Read the model definition and answer for the solid it produces. Units are mm, in the model's axes. A direction names the side the tool comes from. Round coordinates to 2 decimals unless told otherwise and drop trailing zeros. Order: outer loops, then holes, each group sorted by start corner. A loop starts at its lowest first (then second) coordinate and runs counter-clockwise, first axis right, second up. Notation, with made-up numbers: (20.5, 50.5) - (52.5, 50.5) arc R9 cw to (52.5, 65.5) - close; hole circle Ø3 at (-7, 22.5). An arc over 180 degrees is marked (long way). One line per question, with ' | ' between items. Start each with the question number.
1) Flat-ended cylindrical pins translate along their axes: pin 1 (5 mm diameter, centred on y = -81.5, z = 5, fed in from +X); pin 2 (1.5 mm diameter, centred on x = -86, z = 8, fed in from +Y); pin 3 (3 mm diameter, centred on x = 17.5, z = 6, fed in from -Y); pin 4 (3.5 mm diameter, centred on x = -61.35, y = -84.13, fed in from +Z). Find the tip coordinate at first contact, or state that the pin passes through.
2) The part is cut by section D-D, the plane y = 65.5. Give the vertices of the cut face in (x, z), plus the area to 3 significant figures.
3) Straight lines are drawn through the part: line 1 (X direction, y = 6, z = 5.5); line 2 (Y direction, x = -16.5, z = 1); line 3 (X direction, y = 87, z = 4). For each, find the intervals that lie inside material, in ascending order. Write a range as from..to.
4) The mould has two halves that part along Y. Classify faces 4 (the cylindrical face through (-124.84, 5.17, 4.93)), 5 (the flat face through (-41.355, -82, 5)), 6 (the flat face through (58, -96.132, 5)), 7 (the cylindrical face through (-144.84, 7.85, 4.93)): pulls with the +Y half, pulls with the -Y half, needs draft (parallel to the pull), parting line crosses it, or undercut.
5) The part is cut by section B-B, the plane y = 22. Give the vertices of the cut face in (x, z).
6) The part is cut by section A-A, the plane x = 21. Give the vertices of the cut face in (y, z).
7) The part is cut by section C-C, the plane z = 5.25. Give the vertices of the cut face in (x, y), plus the area to 3 significant figures.
8) For faces 1 (the flat face through (78.645, 94, 5)), 2 (the flat face through (-1, 81.068, 5)), 3 (the flat face through (-2, 61.068, 5)), determine the directions among +Z, -Z, +X, -X, +Y, -Y from which every point of the face is accessible in a straight line to the end or side of a thin tool.
from build123d import *

# Parameters (mm, degrees)
SKETCH1_R           = 1.95
BOSS_EXTRUDE1_DEPTH = 10


with BuildPart() as part:
    # Sketch1 → Boss-Extrude1 (new body)
    with BuildSketch(Plane.XY):
        with BuildLine():
            ThreePointArc((-81.354892482, 80.223597026), (-144.854892482, 6.367994666), (-81.354892482, -67.487607695))
            Line((-81.354892482, -67.487607695), (-81.354892482, -96.132005334))
            Line((-81.354892482, -96.132005334), (-41.354892482, -96.132005334))
            Line((-41.354892482, -96.132005334), (-41.354892482, -68.332005334))
            Line((-41.354892482, -68.332005334), (38.645107518, -68.332005334))
            Line((38.645107518, -68.332005334), (38.645107518, -96.132005334))
            Line((38.645107518, -96.132005334), (78.645107518, -96.132005334))
            Line((78.645107518, -96.132005334), (78.645107518, -67.487607695))
            ThreePointArc((78.645107518, -67.487607695), (142.145107518, 6.367994666), (78.645107518, 80.223597026))
            Line((78.645107518, 80.223597026), (78.645107518, 108.867994666))
            Line((78.645107518, 108.867994666), (38.645107518, 108.867994666))
            Line((38.645107518, 108.867994666), (38.645107518, 81.067994666))
            Line((38.645107518, 81.067994666), (-41.354892482, 81.067994666))
            Line((-41.354892482, 81.067994666), (-41.354892482, 108.867994666))
            Line((-41.354892482, 108.867994666), (-81.354892482, 108.867994666))
            Line((-81.354892482, 108.867994666), (-81.354892482, 80.223597026))
        make_face()
        with Locations((-136.354892482, 6.367994666)):
            Circle(SKETCH1_R, mode=Mode.SUBTRACT)
        with Locations((133.645107518, 6.367994666)):
            Circle(SKETCH1_R, mode=Mode.SUBTRACT)
        with BuildLine():
            Line((-70.154892482, 61.067994666), (67.445107518, 61.067994666))
            ThreePointArc((67.445107518, 61.067994666), (122.145107518, 6.367994666), (67.445107518, -48.332005334))
            Line((67.445107518, -48.332005334), (-70.154892482, -48.332005334))
            ThreePointArc((-70.154892482, -48.332005334), (-124.854892482, 6.367994666), (-70.154892482, 61.067994666))
        make_face(mode=Mode.SUBTRACT)
        with Locations((-61.354892482, 96.867994666)):
            Circle(SKETCH1_R, mode=Mode.SUBTRACT)
        with Locations((58.645107518, 96.867994666)):
            Circle(SKETCH1_R, mode=Mode.SUBTRACT)
        with Locations((-61.354892482, -84.132005334)):
            Circle(SKETCH1_R, mode=Mode.SUBTRACT)
        with Locations((58.645107518, -84.132005334)):
            Circle(SKETCH1_R, mode=Mode.SUBTRACT)
    extrude(amount=BOSS_EXTRUDE1_DEPTH)


solid = part.part
Values:
1) pin 1: stops at x = 78.65 | pin 2: stops at y = 79.53 | pin 3: stops at y = -68.33 | pin 4: passes through
2) outline: (-115.8, 0) - (113.09, 0) - (113.09, 10) - (-115.8, 10) - close | area: 2,290 mm^2
3) line 1: x = -144.85..-138.27, -134.44..-124.85, 122.14..131.73, 135.56..142.14 | line 2: y = -68.33..-48.33, 61.07..81.07 | line 3: x = -81.35..-41.35, 38.65..78.65
4) face 4: undercut | face 5: needs draft | face 6: pulls with the -Y half | face 7: parting line crosses it
5) outline: (-143.2, 0) - (-122.57, 0) - (-122.57, 10) - (-143.2, 10) - close; (119.86, 0) - (140.49, 0) - (140.49, 10) - (119.86, 10) - close
6) outline: (-68.33, 0) - (-48.33, 0) - (-48.33, 10) - (-68.33, 10) - close; (61.07, 0) - (81.07, 0) - (81.07, 10) - (61.07, 10) - close
7) outline: (-81.35, -96.13) - (-41.35, -96.13) - (-41.35, -68.33) - (38.65, -68.33) - (38.65, -96.13) - (78.65, -96.13) - (78.65, -67.49) arc R74.7 ccw to (78.65, 80.22) - (78.65, 108.87) - (38.65, 108.87) - (38.65, 81.07) - (-41.35, 81.07) - (-41.35, 108.87) - (-81.35, 108.87) - (-81.35, 80.22) arc R74.7 ccw to (-81.35, -67.49) - close; hole circle Ø3.9 at (-136.35, 6.37); hole (-70.15, -48.33) - (67.45, -48.33) arc R54.7 ccw to (67.45, 61.07) - (-70.15, 61.07) arc R54.7 ccw to start; hole circle Ø3.9 at (-61.35, -84.13); hole circle Ø3.9 at (-61.35, 96.87); hole circle Ø3.9 at (58.65, -84.13); hole circle Ø3.9 at (58.65, 96.87); hole circle Ø3.9 at (133.65, 6.37) | area: 18,000 mm^2
8) face 1: +Z, -Z, +X, +Y | face 2: +Z, -Z, +Y | face 3: +Z, -Z
